Can you work these out from the model? Positions are in its coordinate system, mm. A direction names the side the tool comes from. Coordinates: 2 decimals unless noted, no trailing zeros. Order: outer loops, then holes, each group sorted by start corner. A loop starts at its lowest first (then second) coordinate and runs counter-clockwise, first axis right, second up. Notation, with made-up numbers: (34, 79.5) -> (89, 79.5) arc R17 ccw to (89, 89.5) -> close; hole circle Ø6 at (-11.5, -29.5). An arc over 180 degrees is marked (long way). Write item = value, one per line. Start each with the question number.
from build123d import *

# Parameters (mm, degrees)
F0_W           = 101.6
F0_H           = 101.6
F1_DEPTH       = 12.7
F3_D           = 6.7564
F3_CBORE_D     = 11.176
F3_CBORE_DEPTH = 6.35
F5_D           = 5.1054


with BuildPart() as f1:
    # F0 (on Top) → F1 (new body)
    with BuildSketch(Plane.XY):
        with Locations((-0.288248, -12.711609)):
            Rectangle(F0_W, F0_H)
    extrude(amount=F1_DEPTH)

    # F3 (through all)
    with Locations(Plane.XY.offset(12.7)):
        with Locations((-19.338248, 25.388391), (18.761752, 25.388391), (-19.338248, -50.811609), (18.761752, -50.811609)):
            CounterBoreHole(F3_D / 2, F3_CBORE_D / 2, F3_CBORE_DEPTH)

    # F5 (through all)
    with Locations(Plane.XY.offset(12.7)):
        with Locations((-38.388248, 12.688391), (-38.388248, -38.111609), (37.811752, -38.111609), (37.811752, 12.688391)):
            Hole(F5_D / 2)


solid = f1.part
(1) If I drill on L1, parallel to Y at x = -37, z = 11.75; L2, parallel to X at y = -52, z = 7.5; L3, parallel to Y at x = 39, z = 3.75, over which ranges is the centre line in solid material (lowest first)? Write a range as from..to.
(2) For faces 1 (the face through (-15.7, 25.5, 6.35)), 2 (the face through (-1, 38.088, 6)), which set-ups out of +Z, -Z, +X, -X, +Y, -Y let a thin tool reach every point of the face, with its end or its side?
(3) Imagine slicing it at A-A (x = 17.5). Write out the boundary of the cut face in (y, z).
(4) For P1, Ø4, axis at x = 18.76, y = -50.81, coming from the -Z side; P2, Ø5.5, axis at x = -18, y = 24, coming from the +Z side, each with a flat end and sliding along its axis, tell me the tip position at first contact or that it passes through.
(5) Thinking about a two-plate mould opening in X: for faces 3 (the face through (-51.088, -13, 6)), 4 (the face through (-1, -12, 12.7)), 5 (the face through (50.512, -13, 6)), 6 (the face through (21.34, 20.43, 9.57)), which applies, +X half, -X half, draft (parallel to the pull), parting line (faces both ways), or undercut?
(6) Imagine slicing it at B-B (z = 11.5). Count the separate pieces of the cut face and the enclosed holes in it, plus the area to 3 significant figures.
Result set:
q1.L1 = -63.51..-40.25, -35.97..10.55, 14.83..38.09
q1.L2 = -51.09..-24.8, -13.88..13.3, 24.22..50.51
q1.L3 = -63.51..-40.37, -35.85..10.43, 14.95..38.09
q2.face_1 = +Z
q2.face_2 = +Z, -Z, +X, -X, +Y
q3.outline = (-63.51, 0) -> (-53.95, 0) -> (-53.95, 6.35) -> (-56.26, 6.35) -> (-56.26, 12.7) -> (-63.51, 12.7) -> close; (-47.68, 0) -> (22.25, 0) -> (22.25, 6.35) -> (19.94, 6.35) -> (19.94, 12.7) -> (-45.37, 12.7) -> (-45.37, 6.35) -> (-47.68, 6.35) -> close; (28.52, 0) -> (38.09, 0) -> (38.09, 12.7) -> (30.83, 12.7) -> (30.83, 6.35) -> (28.52, 6.35) -> close
q4.P1 = through
q4.P2 = 6.35
q5.face_3 = -X half
q5.face_4 = draft
q5.face_5 = +X half
q5.face_6 = undercut
q6.separate_pieces = 1
q6.enclosed_holes = 8
q6.area = 9,850 mm2
